Can you work these out from the model? Positions are in its coordinate system, mm. A direction names the side the tool comes from. Give positions to 0.01 mm unless a question says otherwise; leave off trailing zeros. Loops run counter-clockwise (first coordinate to the right, second up) from the corner with the lowest first, then second, coordinate; pieces in that order, holes last. Notation, with made-up numbers: M 28.25,-12 L 62.25,-12 A7 ccw 62.25,-3 Z; hole C -28.5,29 d8. An arc over 180 degrees is marked long. Answer as a JSON object with one key per item and string values.
```python
from build123d import *

# Parameters (mm, degrees)
BOSS_EXTRUDE1_DEPTH = 5
SKETCH2_R           = 20
CUT_EXTRUDE1_DEPTH  = 6
SKETCH3_R           = 30
CUT_EXTRUDE2_DEPTH  = 2
SKETCH4_R           = 2.5
SKETCH4_R_2         = 19.05
CUT_EXTRUDE3_DEPTH  = 6


with BuildPart() as part:
    # Sketch1 → Boss-Extrude1 (new body)
    with BuildSketch(Plane(origin=(0, 0, 0), x_dir=(1, 0, 0), z_dir=(0, 1, 0))):
        with BuildLine():
            ThreePointArc((-110, 53), (-163, 0), (-110, -53))
            Line((-110, -53), (-110, 53))
        make_face()
        with BuildLine():
            Line((-110, 53), (-110, -53))
            ThreePointArc((-110, -53), (-72.523340597, -37.476659403), (-57, 0))
            ThreePointArc((-57, 0), (-72.523340597, 37.476659403), (-110, 53))
        make_face()
        with BuildLine():
            ThreePointArc((-57, 0), (-72.523340597, -37.476659403), (-110, -53))
            Line((-110, -53), (110, -53))
            ThreePointArc((110, -53), (57, 0), (110, 53))
            Line((110, 53), (-110, 53))
            ThreePointArc((-110, 53), (-72.523340597, 37.476659403), (-57, 0))
        make_face()
        with BuildLine():
            ThreePointArc((110, 53), (57, 0), (110, -53))
            Line((110, -53), (110, 53))
        make_face()
        with BuildLine():
            Line((110, 53), (110, -53))
            ThreePointArc((110, -53), (147.476659403, -37.476659403), (163, 0))
            ThreePointArc((163, 0), (147.476659403, 37.476659403), (110, 53))
        make_face()
    extrude(amount=BOSS_EXTRUDE1_DEPTH)

    # Sketch2 → Cut-Extrude1 (cut, through all)
    with BuildSketch(Plane(origin=(0, 5, 0), x_dir=(1, 0, 0), z_dir=(0, 1, 0))):
        with Locations((110, 0)):
            Circle(SKETCH2_R)
    extrude(amount=-CUT_EXTRUDE1_DEPTH, mode=Mode.SUBTRACT)

    # Sketch3 → Cut-Extrude2 (cut)
    with BuildSketch(Plane.XZ):
        with Locations((110, 0)):
            Circle(SKETCH3_R)
    extrude(amount=-CUT_EXTRUDE2_DEPTH, mode=Mode.SUBTRACT)

    # Sketch4 → Cut-Extrude3 (cut, through all)
    with BuildSketch(Plane(origin=(0, 5, 0), x_dir=(1, 0, 0), z_dir=(0, 1, 0))):
        with Locations((-113.57, 23.57)):
            Circle(SKETCH4_R)
        with Locations((-66.43, 23.57)):
            Circle(SKETCH4_R)
        with Locations((-66.43, -23.57)):
            Circle(SKETCH4_R)
        with Locations((-113.57, -23.57)):
            Circle(SKETCH4_R)
        with Locations((-90, 0)):
            Circle(SKETCH4_R_2)
        with BuildLine():
            Line((45.182638641, 10), (45.182638641, 30))
            ThreePointArc((45.182638641, 30), (42.682638641, 32.5), (40.182638641, 30))
            Line((40.182638641, 30), (40.182638641, 10))
            ThreePointArc((40.182638641, 10), (42.682638641, 7.5), (45.182638641, 10))
        make_face()
        with BuildLine():
            Line((40.182638641, -10), (40.182638641, -30))
            ThreePointArc((40.182638641, -30), (42.682638641, -32.5), (45.182638641, -30))
            Line((45.182638641, -30), (45.182638641, -10))
            ThreePointArc((45.182638641, -10), (42.682638641, -7.5), (40.182638641, -10))
        make_face()
    extrude(amount=-CUT_EXTRUDE3_DEPTH, mode=Mode.SUBTRACT)


solid = part.part
```
1) Will these pins go through, and if not, where does the flat tip stop? pin 1 Ø1.5 at (y, z) = (3, -22) entering from +X; pin 2 Ø2.5 at (y, z) = (3, 16) entering from +X; pin 3 Ø1.5 at (y, z) = (1.5, -18.5) entering from -X.
Answer list:
{"pin 1": "x = 158.55", "pin 2": "x = 160.91", "pin 3": "x = -159.94"}
2) For faces 4 (the cylindrical face through (-109.03, 2.54, -0.84)), 5 (the flat face through (130, 2, -6)), which set-ups out of +Z, -Z, +X, -X, +Y, -Y let a thin tool reach every point of the face, with its end or its side?
Answer list:
{"face 4": "+Y, -Y", "face 5": "-Y"}
3) Suppose I cut it at C-C, the plane x = 95. Write out the boundary of the cut face in (y, z).
Answer list:
{"outline": "M 0,-53 L 5,-53 L 5,-13.23 L 2,-13.23 L 2,-25.98 L 0,-25.98 Z; M 0,25.98 L 2,25.98 L 2,13.23 L 5,13.23 L 5,53 L 0,53 Z"}
4) Suppose I cut it at D-D, the plane z = 37.5. Write out the boundary of the cut face in (x, y), and give its area (3 significant figures).
Answer list:
{"outline": "M -147.45,0 L 147.45,0 L 147.45,5 L -147.45,5 Z", "area": "1,470 mm^2"}
5) Suppose I cut it at A-A, the plane x = -90. Write out the boundary of the cut face in (y, z), and give its area (4 significant figures).
Answer list:
{"outline": "M 0,-53 L 5,-53 L 5,-19.05 L 0,-19.05 Z; M 0,19.05 L 5,19.05 L 5,53 L 0,53 Z", "area": "339.5 mm^2"}
6) Suppose I cut it at B-B, the plane y = 3.3. Give the number of separate pieces and of enclosed holes in the cut face, and give its area (3 significant figures).
Answer list:
{"separate pieces": "1", "enclosed holes": "8", "area": "29,400 mm^2"}
7) If we mould it in two halves opening along Z, with no side actions, what happens to faces 1 (the cylindrical face through (90.02, 3.52, -0.88)), 2 (the cylindrical face through (-162.987, 2.465, -1.165)), 3 (the flat face through (-2, 5, -1))? For each: +Z half, -Z half, draft (parallel to the pull), parting line (faces both ways), or undercut.
Answer list:
{"face 1": "undercut", "face 2": "parting line", "face 3": "draft"}
8) Please list where these lines run through material, in increasing order: line 1 along X through (y, z) = (3.9, 1); line 2 along X through (y, z) = (4.1, 11.5); line 3 along X through (y, z) = (3.55, 23.57). Write a range as from..to.
Answer list:
{"line 1": "-162.99..-109.02, -70.98..90.03, 129.97..162.99", "line 2": "-161.74..-105.19, -74.81..40.18, 45.18..93.64, 126.36..161.74", "line 3": "-157.47..-116.07, -111.07..-68.93, -63.93..40.18, 45.18..157.47"}
